Verification items for the finished model (mm, model axes). A direction names the side the tool comes from. Round coordinates to 2 decimals unless told otherwise and drop trailing zeros. Write each loop counter-clockwise with the first axis right and the second up, starting at its lowest first coordinate (ties: lowest second). Pieces come first, ordered by that corner, then holes. Notation, with made-up numbers: (-9, 78.5) -> (30, 78.5) arc R11 ccw to (30, 82.5) -> close; hole circle Ø3 at (77, -15.5). An arc over 180 degrees is marked (long way). Answer as a JSON object with one key per item and string values. Group by question number.
(1) Draft check along Z on faces 1 (the face through (31, -24, -20)), 2 (the face through (31, -39, -24)), 3 (the face through (31, -36, -21)). Enter one of: released by +Z, released by -Z, zero draft, split by the parting line, or undercut.
(2) Sectioned sample at C-C on y = -18.5. Record the cut outline in (x, z), and give its area (3 significant figures).
(3) Gauge pin test, flat ends, axial feed: pin 1 Ø1 at (y, z) = (-36.5, -23.5) entering from +X; pin 2 Ø2.5 at (x, z) = (31, -24) entering from +Y; pin 3 Ø4 at (x, y) = (28.5, -33.5) entering from -Z. Record the tip position at first contact, or that the pin passes through.
(4) Sectioned sample at A-A on z = -24. Record the cut outline in (x, y).
(5) Scan lines: L1, parallel to Z at x = 31, y = -41.5; L2, parallel to X at y = -42.8, z = -24; L3, parallel to Z at x = 32, y = -12. Record each from-to range of solid material in increasing order. Write a range as from..to.
(6) Sectioned sample at D-D on z = -29. Record the cut outline in (x, y).
(7) Sectioned sample at B-B on x = 31. Record the cut outline in (y, z), and give its area (3 significant figures).
(8) Set-up check for faces 4 (the face through (31, -36, -27)), 5 (the face through (27.146, -26.465, -18.101)), 6 (the face through (25.079, -26.465, -20.125)): record each of +Z, -Z, +X, -X, +Y, -Y from which the full face is reachable in a straight line by a thin tool's end or side.
```python
from build123d import *

# Parameters (mm, degrees)
PAD001_DEPTH            = 5
PAD002_DEPTH            = 26
PAD003_DEPTH            = 15
SKETCH016_R             = 1.5
POCKET005_DEPTH         = 5
SKETCH015_R             = 1.5
POCKET006_DEPTH         = 5
BODY002_PLACEMENT_ANGLE = 225


with BuildPart() as part:
    # Sketch004 → Pad001 (new body)
    with BuildSketch(Plane.XZ):
        with BuildLine():
            ThreePointArc((5.823017, 1.446538), (-6, 0), (5.823017, -1.446538))
            Line((5.823017, -1.446538), (8, -1.446538))
            Line((8, -1.446538), (8, 1.446538))
            Line((8, 1.446538), (5.823017, 1.446538))
        make_face()
    extrude(amount=PAD001_DEPTH)

    # Sketch005 (on Face5 of Pad001) → Pad002 (join)
    with BuildSketch(Plane(origin=(0, 0, 0), x_dir=(1, 0, 0), z_dir=(0, 1, 0))):
        with BuildLine():
            ThreePointArc((-0.707105, 4.949749), (-3.535534, 3.535535), (-4.949748, 0.707105))
            Line((-4.949748, 0.707105), (0.707107, -4.949746))
            ThreePointArc((0.707107, -4.949746), (3.535533, -3.535533), (4.949747, -0.707107))
            Line((4.949747, -0.707107), (-0.707105, 4.949749))
        make_face()
    extrude(amount=PAD002_DEPTH)

    # Sketch006 (on Face5 of Pad002) → Pad003 (join)
    with BuildSketch(Plane.XZ.offset(5)):
        with BuildLine():
            ThreePointArc((-4.949747, -0.707107), (-3.535534, -3.535534), (-0.707107, -4.949747))
            Line((-0.707107, -4.949747), (4.949748, 0.707105))
            ThreePointArc((4.949748, 0.707105), (3.535535, 3.535533), (0.707107, 4.949747))
            Line((0.707107, 4.949747), (-4.949747, -0.707107))
        make_face()
    extrude(amount=PAD003_DEPTH)

    # Sketch016 (on Face15 of Pad003) → Pocket005 (cut)
    with BuildSketch(Plane(origin=(0, 26, 0), x_dir=(1, 0, 0), z_dir=(0, 1, 0))):
        Circle(SKETCH016_R)
    extrude(amount=-POCKET005_DEPTH, mode=Mode.SUBTRACT)

    # Sketch015 (on Face16 of Pad003) → Pocket006 (cut)
    with BuildSketch(Plane.XZ.offset(20)):
        Circle(SKETCH015_R)
    extrude(amount=-POCKET006_DEPTH, mode=Mode.SUBTRACT)


with BuildPart() as part_1:
    # Body002 placement: moved
    add(part.part.moved(Location((31, -24, -24.000001))).rotate(Axis((31, -24, -24.000001), (0, 1, 0)), BODY002_PLACEMENT_ANGLE))


solid = part_1.part
```
Computed values:
{
 "1": {"face 1": "zero draft", "face 2": "undercut", "face 3": "released by +Z"},
 "2": {"outline": "(27, -27) -> (35, -27) arc R5 ccw to (35, -21) -> (27, -21) arc R5 ccw to start", "area": "56.2 mm2"},
 "3": {"pin 1": "x = 36", "pin 2": "y = -3", "pin 3": "z = -27"},
 "4": {"outline": "(25, -29) -> (26, -29) -> (26, -44) -> (29.5, -44) -> (29.5, -39) -> (32.5, -39) -> (32.5, -44) -> (36, -44) -> (36, -29) -> (37, -29) -> (37, -24) -> (36, -24) -> (36, 2) -> (32.5, 2) -> (32.5, -3) -> (29.5, -3) -> (29.5, 2) -> (26, 2) -> (26, -24) -> (25, -24) -> close"},
 "5": {"L1": "-27..-25.5, -22.5..-21", "L2": "26..29.5, 32.5..36", "L3": "-27..-21"},
 "6": {"outline": "(27.68, -29) -> (34.32, -29) -> (34.32, -24) -> (27.68, -24) -> close"},
 "7": {"outline": "(-44, -27) -> (-29, -27) -> (-29, -30) -> (-24, -30) -> (-24, -27) -> (2, -27) -> (2, -25.5) -> (-3, -25.5) -> (-3, -22.5) -> (2, -22.5) -> (2, -21) -> (-24, -21) -> (-24, -18) -> (-29, -18) -> (-29, -21) -> (-44, -21) -> (-44, -22.5) -> (-39, -22.5) -> (-39, -25.5) -> (-44, -25.5) -> close", "area": "276 mm2"},
 "8": {"face 4": "-Z, +X, -X, -Y", "face 5": "+Z, +Y, -Y", "face 6": "-X, +Y, -Y"}
}
